The model under review builds one solid part; all positions refer to its coordinate system, in mm. A direction names the side the tool comes from. Coordinates: 2 decimals unless noted, no trailing zeros. Order: outer loops, then holes, each group sorted by start corner. A loop starts at its lowest first (then second) coordinate and runs counter-clockwise, first axis right, second up.
```python
from build123d import *

# Parameters (mm, degrees)
PLASTIC_DEPTH   = 2.54
CONTACT_DEPTH   = 0.3
CHAMFER1_SIZE   = 0.1
LPATTERN1_COUNT = 2
LPATTERN1_PITCH = 2.54


with BuildPart() as part:
    # Sketch1 → Plastic (new body)
    with BuildSketch(Plane(origin=(0, 0, 0), x_dir=(0, 0, -1), z_dir=(1, 0, 0))):
        Polygon((-2.04, 1.27), (-0.5, 1.27), (0, 0.77), (0, -0.77), (-0.5, -1.27), (-2.04, -1.27), (-2.54, -0.77), (-2.54, 0.77), align=None)
    extrude(amount=PLASTIC_DEPTH)

    # Sketch2 → Contact (add, symmetric)
    with BuildSketch(Plane(origin=(0, 0, 0), x_dir=(1, 0, 0), z_dir=(0, 1, 0))):
        with BuildLine():
            Line((-1.86, 3.36), (-1.86, -0.67))
            ThreePointArc((-1.86, -0.67), (-1.596396103, -1.306396103), (-0.96, -1.57))
            Line((-0.96, -1.57), (8.9, -1.57))
            Line((8.9, -1.57), (8.9, -0.97))
            Line((8.9, -0.97), (-0.96, -0.97))
            ThreePointArc((-0.96, -0.97), (-1.172132034, -0.882132034), (-1.26, -0.67))
            Line((-1.26, -0.67), (-1.26, 3.36))
            Line((-1.26, 3.36), (-1.86, 3.36))
        make_face()
    extrude(amount=CONTACT_DEPTH, both=True)

    # Chamfer1
    chamfer1_edges = [part.edges().sort_by_distance(p)[0] for p in [
        (8.9, 0, 0.97),
        (8.9, 0.3, 1.27),
        (-1.56, -0.3, -3.36),
        (-1.26, 0, -3.36),
        (-1.86, 0, -3.36),
        (8.9, -0.3, 1.27),
        (8.9, 0, 1.57),
        (-1.56, 0.3, -3.36),
    ]]
    chamfer(chamfer1_edges, length=CHAMFER1_SIZE)

    # LPattern1: part ×2


with BuildPart() as part_1:
    add(part.part)
    with Locations(*[(0, i * LPATTERN1_PITCH, 0) for i in range(1, LPATTERN1_COUNT)]):
        add(part.part)


solid = part_1.part
```
(1) For pin 1 Ø0.5 at (x, z) = (4.5, 1.5) entering from -Y; pin 2 Ø0.7 at (x, y) = (-0.5, 2.5) entering from +Z; pin 3 Ø1.5 at (x, z) = (-1, 0) entering from +Y; pin 4 Ø2 at (x, z) = (0, -2) entering from +Y, all flat-tipped, find the tip position at first contact; note any pin that passes through.
A:
pin 1: stops at y = -0.3
pin 2: stops at z = 1.57
pin 3: stops at y = 2.84
pin 4: passes through
(2) Machinability: for faces 1 (the face through (-1.6, 2.84, -0.3)), 2 (the face through (-1.6, -0.3, -0.3)), 3 (the face through (1, 0, 0)), 4 (the face through (1, 0, 2.54)), which of the approach directions +Z, -Z, +X, -X, +Y, -Y give a long, thin tool a straight path to every point of the face, cutting with its end or side? Answer none if there is none.
A:
face 1: +Z, -Z, -X, +Y
face 2: +Z, -Z, -X, -Y
face 3: -Z, +X, +Y, -Y
face 4: +Z, +X, -X, +Y, -Y
(3) Draft analysis for pull direction Y (two halves, no side actions). For faces 5 (the face through (-1.6, 0.3, -0.3)), 6 (the face through (-1.6, 2.5, 1.3)), 7 (the face through (-1.6, 2.24, -0.3)), 8 (the face through (1, 3.81, 1)), state which applies: released by +Y, released by -Y, zero draft, split by the parting line, or undercut.
A:
face 5: undercut
face 6: zero draft
face 7: undercut
face 8: released by +Y
(4) We need section A-A, the plane z = 0.3. Write out the cut boundary in (x, y).
A:
outline: (-1.86, -0.3) - (-1.26, -0.3) - (-1.26, 0.3) - (-1.86, 0.3) - close; (-1.86, 2.24) - (-1.26, 2.24) - (-1.26, 2.84) - (-1.86, 2.84) - close; (0, -1.07) - (2.54, -1.07) - (2.54, 1.07) - (0, 1.07) - close; (0, 1.47) - (2.54, 1.47) - (2.54, 3.61) - (0, 3.61) - close
(5) We need section B-B, the plane x = -0.5. Write out the cut boundary in (y, z).
A:
outline: (-0.3, 0.97) - (0.3, 0.97) - (0.3, 1.57) - (-0.3, 1.57) - close; (2.24, 0.97) - (2.84, 0.97) - (2.84, 1.57) - (2.24, 1.57) - close
(6) Wall thickness on probe 1 along Z at (x, y) = (0.75, 1.9); probe 2 along Z at (x, y) = (4.25, 2.75); probe 3 along Y at (x, z) = (4.75, 1.4): over which ranges is each line inside the solid? List them lowest first.
A:
probe 1: z = 0 to 2.54
probe 2: z = 0.97 to 1.57
probe 3: y = -0.3 to 0.3, 2.24 to 2.84
(7) We need section D-D, the plane x = 1.75. Write out the cut boundary in (y, z), and give its area (3 significant figures).
A:
outline: (-1.27, 0.5) - (-0.77, 0) - (0.77, 0) - (1.27, 0.5) - (1.77, 0) - (3.31, 0) - (3.81, 0.5) - (3.81, 2.04) - (3.31, 2.54) - (1.77, 2.54) - (1.27, 2.04) - (0.77, 2.54) - (-0.77, 2.54) - (-1.27, 2.04) - close
area: 11.9 mm2
(8) We need section C-C, the plane z = -2.85. Write out the cut boundary in (x, y), and give its area (3 significant figures).
A:
outline: (-1.86, -0.3) - (-1.26, -0.3) - (-1.26, 0.3) - (-1.86, 0.3) - close; (-1.86, 2.24) - (-1.26, 2.24) - (-1.26, 2.84) - (-1.86, 2.84) - close
area: 0.720 mm2
